Check sheet for the drawn part. Datum: minimum x, y, z corner. Units: mm. Give positions to 0.01 mm unless a question says otherwise; leave off trailing zeros. Order: outer loops, then holes, each group sorted by start corner. A loop starts at its lowest first (then second) coordinate and runs counter-clockwise, first axis right, second up. Notation, with made-up numbers: M 28,2 L 77,2 A22 cw 77,11 Z; hole C 17.5,71.5 d11. An arc over 180 degrees is marked long. Put each result on its own line as item: value. Start each with the question number.
Q1. Section check B-B on y = 1.05. Record the cut outline in (x, z).
Q2. Material ranges on L1, parallel to X at y = 1.1, z = 153; L2, parallel to X at y = 0.9, z = 293; L3, parallel to Z at x = 146.5, y = 0.6, recorded low to high.
Q3. Go/stop test with flat-tipped pins: pin 1 (8 mm diameter, centred on x = 113, z = 219, fed in from -Y); pin 2 (1.5 mm diameter, centred on y = 1.5, z = 291.5, fed in from +X); pin 3 (0.9 mm diameter, centred on x = 18, y = 1, fed in from -Z); pin 4 (0.9 mm diameter, centred on y = 1.5, z = 2, fed in from -X). Record where each tip stops, or that it passes through.
Q4. Section check A-A on x = 150. Record the cut outline in (y, z), then the cut area to 3 significant figures.
Q5. Section check D-D on x = 23. Record the cut outline in (y, z).
Q6. Section check C-C on z = 153. Record the cut outline in (x, y).
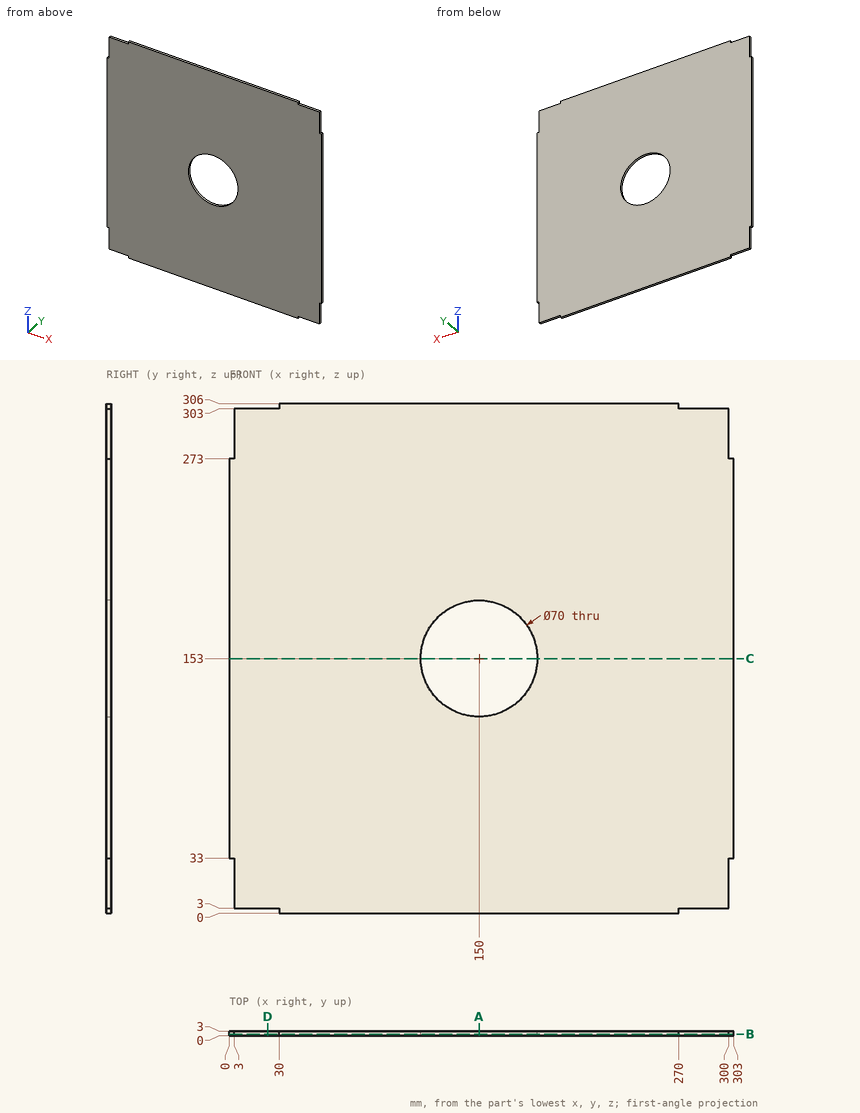
Results found:
1. outline: M 0,33 L 3,33 L 3,3 L 30,3 L 30,0 L 270,0 L 270,3 L 300,3 L 300,33 L 303,33 L 303,273 L 300,273 L 300,303 L 270,303 L 270,306 L 30,306 L 30,303 L 3,303 L 3,273 L 0,273 Z; hole C 150,153 d70
2. L1: x = 0 to 115, 185 to 303
2. L2: x = 3 to 300
2. L3: z = 0 to 118.18, 187.82 to 306
3. pin 1: stops at y = 0
3. pin 2: stops at x = 300
3. pin 3: stops at z = 3
3. pin 4: stops at x = 30
4. outline: M 0,0 L 3,0 L 3,118 L 0,118 Z; M 0,188 L 3,188 L 3,306 L 0,306 Z
4. area: 708 mm^2
5. outline: M 0,3 L 3,3 L 3,303 L 0,303 Z
6. outline: M 0,0 L 115,0 L 115,3 L 0,3 Z; M 185,0 L 303,0 L 303,3 L 185,3 Z
